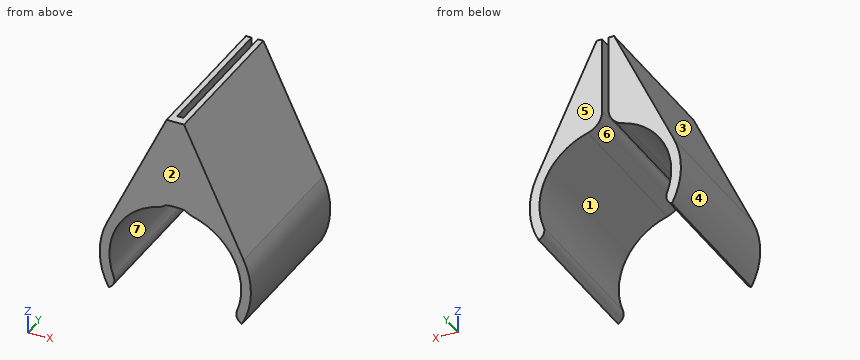
```python
from build123d import *

# Parameters (mm, degrees)
FIN_SLOT_EXTRUDE_DEPTH = 80
FIN_START              = -75
FIN_SLOT_DEPTH         = 75
FILLET1_R              = 10
FILLET2_R              = 5


with BuildPart() as part:
    # Sketch2 → Fin slot extrude (new body)
    with BuildSketch(Plane(origin=(0, 0, 0), x_dir=(1, 0, 0), z_dir=(0, 1, 0))):
        with BuildLine():
            Line((-35.253910446, -16.678183302), (-4.5, -81.685))
            Line((-4.5, -81.685), (4.5, -81.685))
            Line((4.5, -81.685), (35.253910446, -16.678183302))
            ThreePointArc((35.253910446, -16.678183302), (38.987980591, 0.968178408), (34.382638025, 18.407449646))
            Line((34.382638025, 18.407449646), (30.049957519, 15.90597539))
            ThreePointArc((30.049957519, 15.90597539), (0, -34), (-30.049957519, 15.90597539))
            Line((-30.049957519, 15.90597539), (-34.382638025, 18.407449646))
            ThreePointArc((-34.382638025, 18.407449646), (-38.987980591, 0.968178408), (-35.253910446, -16.678183302))
        make_face()
    extrude(amount=FIN_SLOT_EXTRUDE_DEPTH)

    # Sketch3 → Fin slot (cut)
    with BuildSketch(Plane(origin=(0, 80, 0), x_dir=(1, 0, 0), z_dir=(0, 1, 0)).offset(FIN_START)):
        with BuildLine():
            Line((1.6, -81.685), (1.6, -33.962332075))
            ThreePointArc((1.6, -33.962332075), (0, -34), (-1.6, -33.962332075))
            Line((-1.6, -33.962332075), (-1.6, -81.685))
            Line((-1.6, -81.685), (1.6, -81.685))
        make_face()
    extrude(amount=FIN_SLOT_DEPTH, mode=Mode.SUBTRACT)

    # Fillet1
    # the kernel refuses this fillet: 10 mm, written as the material it takes off along each edge
    with BuildSketch(Plane(origin=(-1.6, 5, 33.962332075), x_dir=(0, 0, 1), z_dir=(0, 1, 0))) as fillet1_piece_1:
        with BuildLine():
            CenterArc((8.481041966, -10), FILLET1_R, 90, 74.714058958)
            Line((-1.165179407, -7.363636364), (-1.358103835, -7.310909091))
            ThreePointArc((-1.358103835, -7.310909091), (-0.577691759, -3.682593204), (-0.199778424, 0.009411765))
            Line((-0.199778424, 0.009411765), (0, 0.2))
            Line((0, 0.2), (8.481041966, 0.2))
            Line((8.481041966, 0.2), (8.481041966, 0))
        make_face()
    extrude(amount=75, mode=Mode.SUBTRACT)
    with BuildSketch(Plane(origin=(1.6, 5, 33.962332075), x_dir=(0, 0, 1), z_dir=(0, 1, 0))) as fillet1_piece_2:
        with BuildLine():
            CenterArc((8.481041966, 10), FILLET1_R, 195.285941042, 74.714058958)
            Line((-1.165179407, 7.363636364), (-1.358103835, 7.310909091))
            ThreePointArc((-1.358103835, 7.310909091), (-0.577691759, 3.682593204), (-0.199778424, -0.009411765))
            Line((-0.199778424, -0.009411765), (0, -0.2))
            Line((0, -0.2), (8.481041966, -0.2))
            Line((8.481041966, -0.2), (8.481041966, 0))
        make_face()
    extrude(amount=75, mode=Mode.SUBTRACT)
    with BuildSketch(Plane(origin=(0, 5, 0), x_dir=(0.7049632922211216, 0, 0.7092437920918008), z_dir=(0.7092437920918008, 0, -0.7049632922211216))) as fillet1_piece_3_section:
        with BuildLine():
            CenterArc((34 + FILLET1_R, FILLET1_R), FILLET1_R, 180, 90)
            Line((34, FILLET1_R), (34 - FILLET1_R * 0.02, FILLET1_R))
            Line((34 - FILLET1_R * 0.02, FILLET1_R), (34 - FILLET1_R * 0.02, -FILLET1_R * 0.02))
            Line((34 - FILLET1_R * 0.02, -FILLET1_R * 0.02), (34 + FILLET1_R, -FILLET1_R * 0.02))
            Line((34 + FILLET1_R, -FILLET1_R * 0.02), (34 + FILLET1_R, 0))
        make_face()
    fillet1_piece_3 = revolve(axis=Axis((0, 5, 0), (0, -1, 0)), revolution_arc=89.653157122, mode=Mode.PRIVATE)
    fillet1_piece_3 = split(fillet1_piece_3, bisect_by=Plane(origin=(1.6, 2.736001805, 36.252063161), z_dir=(-1, 0, 0)), keep=Keep.TOP, mode=Mode.PRIVATE)
    fillet1_piece_3 = split(fillet1_piece_3, bisect_by=Plane(origin=(-1.6, 2.736001805, 36.252063161), z_dir=(1, 0, 0)), keep=Keep.TOP, mode=Mode.PRIVATE)
    add(fillet1_piece_3, mode=Mode.SUBTRACT)
    with BuildSketch(Plane(origin=(0, 5, 0), x_dir=(0.7049632922211216, 0, 0.7092437920918008), z_dir=(0.7092437920918008, 0, -0.7049632922211216))) as fillet1_piece_4a_section:
        with BuildLine():
            CenterArc((34 + FILLET1_R, FILLET1_R), FILLET1_R, 180, 90)
            Line((34, FILLET1_R), (34 - FILLET1_R * 0.02, FILLET1_R))
            Line((34 - FILLET1_R * 0.02, FILLET1_R), (34 - FILLET1_R * 0.02, -FILLET1_R * 0.02))
            Line((34 - FILLET1_R * 0.02, -FILLET1_R * 0.02), (34 + FILLET1_R, -FILLET1_R * 0.02))
            Line((34 + FILLET1_R, -FILLET1_R * 0.02), (34 + FILLET1_R, 0))
        make_face()
    fillet1_piece_4a = revolve(axis=Axis((0, 5, 0), (0, -1, 0)), revolution_arc=89.653157122, mode=Mode.PRIVATE)
    fillet1_piece_4a = split(fillet1_piece_4a, bisect_by=Plane(origin=(-1.6, 2.81629174, 32.584573329), z_dir=(-1, 0, 0)), keep=Keep.TOP, mode=Mode.PRIVATE)
    with BuildSketch(Plane(origin=(-1.6, -16.202604914, 33.962332075), x_dir=(0, 0, 1), z_dir=(0, 1, 0))) as fillet1_piece_4b_section:
        with BuildLine():
            CenterArc((8.481041966, -10), FILLET1_R, 90, 74.714058958)
            Line((-1.165179407, -7.363636364), (-1.358103835, -7.310909091))
            ThreePointArc((-1.358103835, -7.310909091), (-0.577691759, -3.682593204), (-0.199778424, 0.009411765))
            Line((-0.199778424, 0.009411765), (0, 0.2))
            Line((0, 0.2), (8.481041966, 0.2))
            Line((8.481041966, 0.2), (8.481041966, 0))
        make_face()
    fillet1_piece_4b = extrude(amount=96.202604914, mode=Mode.PRIVATE)
    fillet1_piece_4b = split(fillet1_piece_4b, bisect_by=Plane(origin=(-3.235617235, 5, 35.755925785), z_dir=(0, -1, 0)), keep=Keep.TOP, mode=Mode.PRIVATE)
    fillet1_piece_4 = fillet1_piece_4a & fillet1_piece_4b
    add(fillet1_piece_4, mode=Mode.SUBTRACT)
    with BuildSketch(Plane(origin=(1.6, -16.202604914, 33.962332075), x_dir=(0, 0, 1), z_dir=(0, 1, 0))) as fillet1_piece_5a_section:
        with BuildLine():
            CenterArc((8.481041966, 10), FILLET1_R, 195.285941042, 74.714058958)
            Line((-1.165179407, 7.363636364), (-1.358103835, 7.310909091))
            ThreePointArc((-1.358103835, 7.310909091), (-0.577691759, 3.682593204), (-0.199778424, -0.009411765))
            Line((-0.199778424, -0.009411765), (0, -0.2))
            Line((0, -0.2), (8.481041966, -0.2))
            Line((8.481041966, -0.2), (8.481041966, 0))
        make_face()
    fillet1_piece_5a = extrude(amount=96.202604914, mode=Mode.PRIVATE)
    fillet1_piece_5a = split(fillet1_piece_5a, bisect_by=Plane(origin=(3.235617235, 5, 35.755925785), z_dir=(0, -1, 0)), keep=Keep.TOP, mode=Mode.PRIVATE)
    with BuildSketch(Plane(origin=(0, 5, 0), x_dir=(0.7049632922211216, 0, 0.7092437920918008), z_dir=(0.7092437920918008, 0, -0.7049632922211216))) as fillet1_piece_5b_section:
        with BuildLine():
            CenterArc((34 + FILLET1_R, FILLET1_R), FILLET1_R, 180, 90)
            Line((34, FILLET1_R), (34 - FILLET1_R * 0.02, FILLET1_R))
            Line((34 - FILLET1_R * 0.02, FILLET1_R), (34 - FILLET1_R * 0.02, -FILLET1_R * 0.02))
            Line((34 - FILLET1_R * 0.02, -FILLET1_R * 0.02), (34 + FILLET1_R, -FILLET1_R * 0.02))
            Line((34 + FILLET1_R, -FILLET1_R * 0.02), (34 + FILLET1_R, 0))
        make_face()
    fillet1_piece_5b = revolve(axis=Axis((0, 5, 0), (0, -1, 0)), revolution_arc=89.653157122, mode=Mode.PRIVATE)
    fillet1_piece_5b = split(fillet1_piece_5b, bisect_by=Plane(origin=(1.6, 2.816291902, 32.584573464), z_dir=(1, 0, 0)), keep=Keep.TOP, mode=Mode.PRIVATE)
    fillet1_piece_5 = fillet1_piece_5a & fillet1_piece_5b
    add(fillet1_piece_5, mode=Mode.SUBTRACT)

    # Fillet2
    fillet2_edges = [part.edges().sort_by_distance(p)[0] for p in [
        (-30.049957519, 40, -15.90597539),
        (30.049957519, 40, -15.90597539),
    ]]
    fillet(fillet2_edges, radius=FILLET2_R)


solid = part.part
```
Part model, mm, in its own coordinate system. Face numbers are marked on the shaded views. A direction names the side the tool comes from. Round coordinates to 2 decimals unless told otherwise and drop trailing zeros. Write each loop counter-clockwise with the first axis right and the second up, starting at its lowest first coordinate (ties: lowest second). Pieces come first, ordered by that corner, then holes. Notation, with made-up numbers: (-36, -27.5) -> (-18, -27.5) arc R20 cw to (-18, -22.5) -> close; hole circle Ø1 at (34, -23). An arc over 180 degrees is marked (long way). Return JSON: item names as keys, results as strings. Group by question number.
Q1. Saw through at B-B on y = 63.5. Write the cut outline in (x, z) (3 decimals).
Q2. Saw through at D-D on z = 61. Write the cut outline in (x, y).
Q3. Mould opens along Z. For the marked faces 1, 2, 3 and 4 say: pulls with the +Z half, pulls with the -Z half, needs draft (parallel to the pull), parting line crosses it, or undercut.
Q4. Saw through at C-C on z = -4.5. Write the cut outline in (x, y), plus the area to 3 significant figures.
Q5. Saw through at A-A on z = 20.5. Write the cut outline in (x, y), plus the area to 3 significant figures.
Q6. Pin check, flat tips, straight feed: pin 1 (2.5 mm diameter, centred on x = 0, z = 61.5, fed in from +Y); pin 2 (1 mm diameter, centred on x = -23.5, y = 16, fed in from -Z); pin 3 (6 mm diameter, centred on y = 34.5, z = 64, fed in from -X). Stop position of each tip, or through.
Q7. Which spindle directions (+Z, -Z, +X, -X, +Y, -Y) get a long thin tool onto all of the face, cutting with end or side? Do the marked faces 5, 6 and 7. Say none if no direction does.
Q8. Probe L1, parallel to X at y = 37, z = -1; L2, parallel to X at y = 8.5, z = -4.5; L3, parallel to Z at x = -14.5, y = 20. List the from-to ranges inside material, lowest first. Write a range as [from, to].
Answer:
{
 "1": {"outline": "(-35.254, 16.678) arc R39 ccw to (-34.383, -18.407) -> (-33.963, -18.165) arc R5 ccw to (-31.789, -12.062) arc R34 cw to (-8.964, 32.797) arc R10 ccw to (-1.6, 42.443) -> (-1.6, 81.685) -> (-4.5, 81.685) -> close; (1.6, 42.443) arc R10 ccw to (8.964, 32.797) arc R34 cw to (31.789, -12.062) arc R5 ccw to (33.963, -18.165) -> (34.383, -18.407) arc R39 ccw to (35.254, 16.678) -> (4.5, 81.685) -> (1.6, 81.685) -> close"},
 "2": {"outline": "(-14.29, 0) -> (14.29, 0) -> (14.29, 80) -> (1.6, 80) -> (1.6, 5) -> (-1.6, 5) -> (-1.6, 80) -> (-14.29, 80) -> close"},
 "3": {"face 1": "undercut", "face 2": "needs draft", "face 3": "pulls with the +Z half", "face 4": "parting line crosses it"},
 "4": {"outline": "(-38.74, 0) -> (-33.7, 0) -> (-33.7, 80) -> (-38.74, 80) -> close; (33.7, 0) -> (38.74, 0) -> (38.74, 80) -> (33.7, 80) -> close", "area": "806 mm2"},
 "5": {"outline": "(-33.45, 0) -> (-27.12, 0) -> (-27.12, 80) -> (-33.45, 80) -> close; (27.12, 0) -> (33.45, 0) -> (33.45, 80) -> (27.12, 80) -> close", "area": "1,010 mm2"},
 "6": {"pin 1": "y = 5", "pin 2": "z = 24.08", "pin 3": "x = -14.29"},
 "7": {"face 5": "+Z, -Z, +X, -X, +Y", "face 6": "-Z, +Y", "face 7": "+Y, -Y"},
 "8": {"L1": "[-38.99, -33.99], [33.99, 38.99]", "L2": "[-38.74, -33.7], [33.7, 38.74]", "L3": "[30.75, 60.55]"}
}
